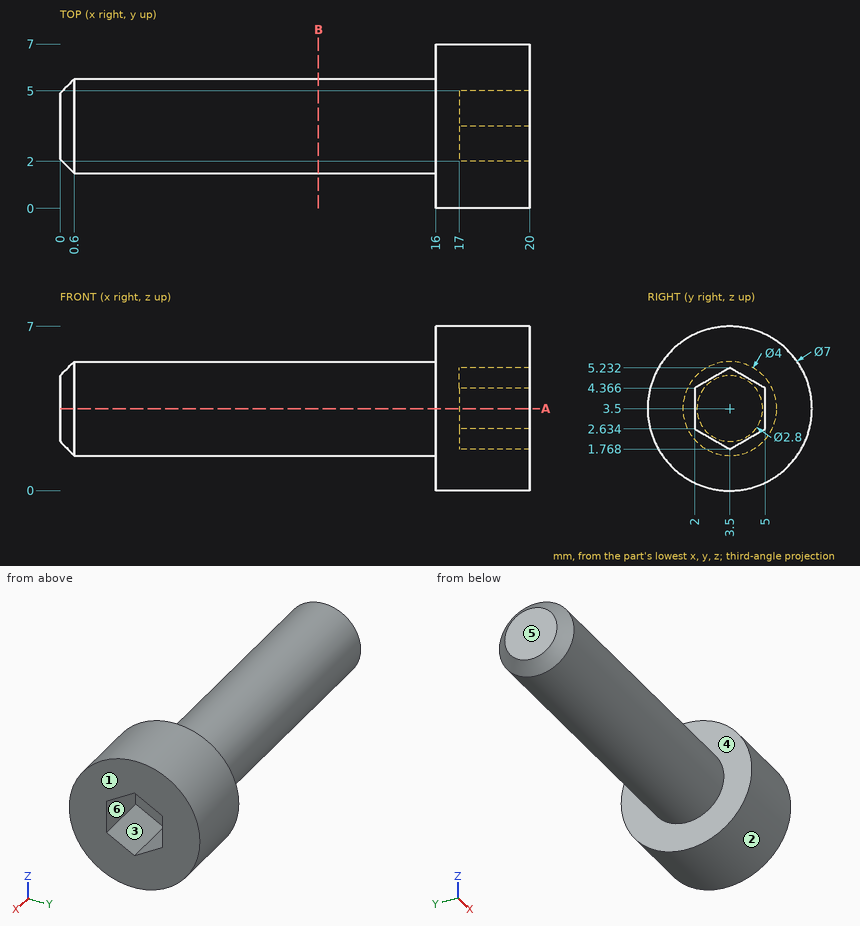
Answer from the drawing. Dimensions are ordinates in mm from the lowest x, y and z of the part. A direction names the side the tool comes from. Give positions to 0.01 mm unless a question says otherwise; leave off trailing zeros. Order: outer loops, then holes, each group sorted by start corner. A loop starts at its lowest first (then second) coordinate and runs counter-clockwise, first axis right, second up. Notation, with made-up numbers: (26.25, 68) -> (76.25, 68) arc R33 ccw to (76.25, 106) -> close; hole circle Ø10 at (84, -7.5). An arc over 180 degrees is marked (long way). Answer as a JSON object with one key per item and string values. Group by question number.
1. Section B-B on x = 11 is taken. Determine the outline of the cut face in (y, z), plus the area to 3 significant figures.
2. Flat-ended cylindrical pins translate along their axes: pin 1 Ø1 at (x, z) = (2.5, 2) entering from -Y; pin 2 Ø3 at (x, y) = (6.5, 2.5) entering from -Z; pin 3 Ø2 at (y, z) = (2, 6) entering from -X. Find the tip coordinate at first contact, or state that the pin passes through.
3. The mould has two halves that part along Y. Classify the marked faces 1, 2 and 3: released by +Y, released by -Y, zero draft, split by the parting line, or undercut.
4. A tool of negligible diameter and unlimited length cuts with its end or side. For the marked faces 4, 5 and 6, from which of +Z, -Z, +X, -X, +Y, -Y can it reach the whole face along a straight path? Write none if from no direction.
5. Consider line 1 along X through (y, z) = (6.5, 2.75); line 2 along X through (y, z) = (2.5, 4); line 3 along Y through (x, z) = (19, 4.75) (1 decimal). Determine where each line is inside the solid, lowest interval first. Write a range as [from, to].
6. Section A-A on z = 3.5 is taken. Determine the outline of the cut face in (x, y).
Result sheet:
{
 "1": {"outline": "circle Ø4 at (3.5, 3.5)", "area": "12.6 mm^2"},
 "2": {"pin 1": "stops at y = 1.77", "pin 2": "stops at z = 1.5", "pin 3": "stops at x = 0.52"},
 "3": {"face 1": "zero draft", "face 2": "split by the parting line", "face 3": "undercut"},
 "4": {"face 4": "-X", "face 5": "+Z, -Z, -X, +Y, -Y", "face 6": "+X"},
 "5": {"line 1": "x = [16, 20]", "line 2": "x = [0, 17]", "line 3": "y = [0.2, 2.7], [4.3, 6.8]"},
 "6": {"outline": "(0, 2.1) -> (0.6, 1.5) -> (16, 1.5) -> (16, 0) -> (20, 0) -> (20, 2) -> (17, 2) -> (17, 5) -> (20, 5) -> (20, 7) -> (16, 7) -> (16, 5.5) -> (0.6, 5.5) -> (0, 4.9) -> close"}
}
